Geometry check sheet. Reference: drawing and pictorial views, mm from the part's lowest x, y, z. A direction names the side the tool comes from. Give positions to 0.01 mm unless a question says otherwise; leave off trailing zeros. Order: outer loops, then holes, each group sorted by start corner. A loop starts at its lowest first (then second) coordinate and runs counter-clockwise, first axis right, second up.
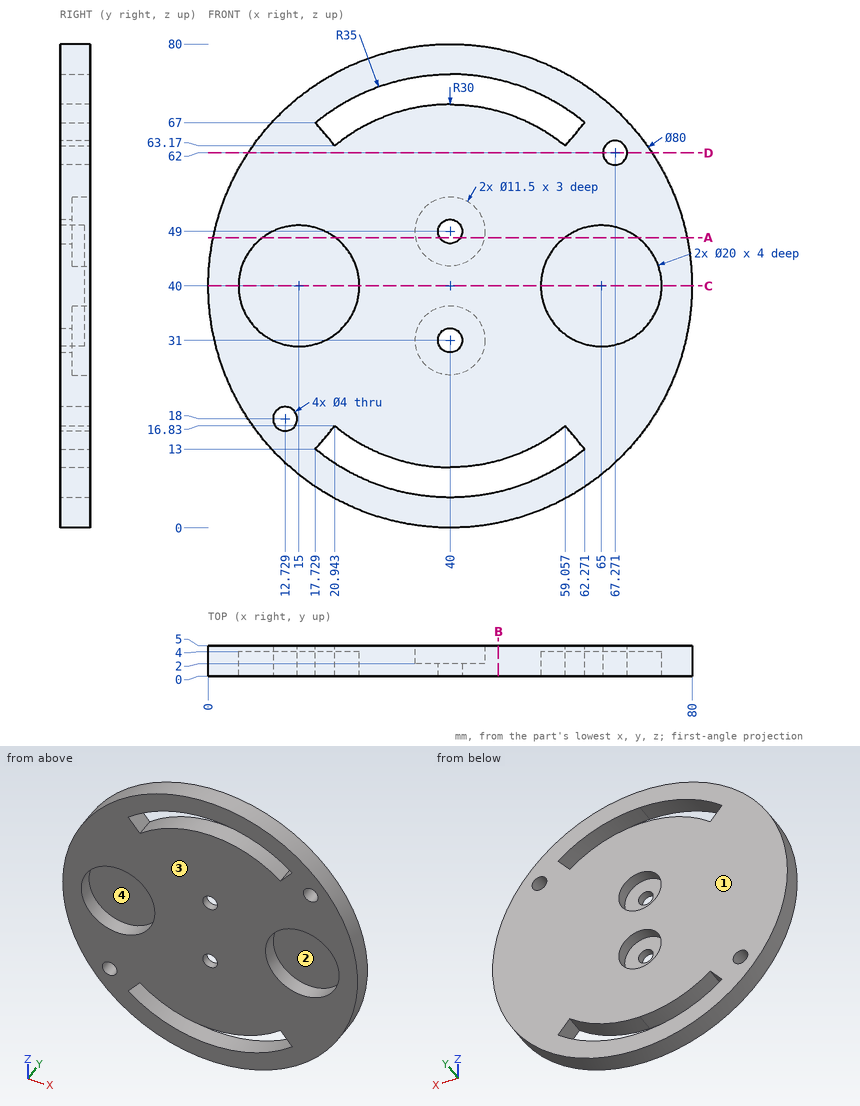
1) Depth check by flat-ended pin: pin 1 Ø3 at (x, y) = (27.5, 1) entering from +Z; pin 2 Ø6 at (x, z) = (38, 49.5) entering from +Y; pin 3 Ø6 at (x, z) = (65, 44) entering from -Y. Enter the tip coordinate at first touch or a pass-through.
Recorded:
pin 1: stops at z = 78.46
pin 2: stops at y = 2
pin 3: stops at y = 4
2) Section check C-C, the plane z = 40. Record the cut outline in (x, y), then the cut area to 3 significant figures.
Recorded:
outline: (0, 0) - (5, 0) - (5, 4) - (25, 4) - (25, 0) - (55, 0) - (55, 4) - (75, 4) - (75, 0) - (80, 0) - (80, 5) - (0, 5) - close
area: 240 mm2
3) Section check D-D, the plane z = 62. Record the cut outline in (x, y), then the cut area to 3 significant figures.
Recorded:
outline: (6.59, 0) - (65.27, 0) - (65.27, 5) - (6.59, 5) - close; (69.27, 0) - (73.41, 0) - (73.41, 5) - (69.27, 5) - close
area: 314 mm2
4) Section check A-A, the plane z = 48. Record the cut outline in (x, y).
Recorded:
outline: (0.81, 0) - (9, 0) - (9, 4) - (21, 4) - (21, 0) - (38.27, 0) - (38.27, 2) - (34.34, 2) - (34.34, 5) - (0.81, 5) - close; (41.73, 0) - (59, 0) - (59, 4) - (71, 4) - (71, 0) - (79.19, 0) - (79.19, 5) - (45.66, 5) - (45.66, 2) - (41.73, 2) - close
5) Section check B-B, the plane x = 48. Record the cut outline in (y, z).
Recorded:
outline: (0, 0.81) - (5, 0.81) - (5, 5.93) - (0, 5.93) - close; (0, 11.09) - (5, 11.09) - (5, 68.91) - (0, 68.91) - close; (0, 74.07) - (5, 74.07) - (5, 79.19) - (0, 79.19) - close
6) Material ranges on L1, parallel to X at y = 3.35, z = 13 (1 decimal); L2, parallel to Z at x = 35, y = 4.4 (1 decimal); L3, parallel to X at y = 1.3, z = 31.5 (1 decimal), recorded low to high.
Recorded:
L1: x = 10.5 to 17.7, 26.9 to 53.1, 62.3 to 69.5
L2: z = 0.3 to 5.4, 10.4 to 28.2, 33.8 to 46.2, 51.8 to 69.6, 74.6 to 79.7
L3: x = 0.9 to 9.7, 20.3 to 38.1, 41.9 to 59.7, 70.3 to 79.1
7) Draft check along Z on the marked faces 1 and 2. Enter one of: +Z half, -Z half, draft (parallel to the pull), parting line (faces both ways), or undercut.
Recorded:
face 1: draft
face 2: undercut
8) Set-up check for the marked faces 3 and 4: record each of +Z, -Z, +X, -X, +Y, -Y from which the full face is reachable in a straight line by a thin tool's end or side.
Recorded:
face 3: +Z, -Z, +X, -X, -Y
face 4: -Y
